Geometry check sheet. Reference: the model listing, model coordinates, mm. Face numbers are marked on the shaded views. A direction names the side the tool comes from. Give positions to 0.01 mm unless a question says otherwise; leave off trailing zeros. Order: outer loops, then holes, each group sorted by start corner. A loop starts at its lowest first (then second) coordinate and runs counter-clockwise, first axis right, second up. Notation, with made-up numbers: M -19,2 L -2,2 A7 cw -2,11 Z; hole C 1.25,26.25 d3. An arc over 180 degrees is marked long. Put each result on its own line as item: value. Start each with the question number.
Q1. Mould release check, pull along X, two halves, no side actions. Record for the marked faces 1, 2 and 3: +X half, -X half, draft (parallel to the pull), parting line (faces both ways), or undercut.
Q2. Material ranges on L1, parallel to Y at x = -0.5, z = -0.7; L2, parallel to Y at x = 0.25, z = 1.75; L3, parallel to X at y = 4, z = 0.65, recorded low to high.
Q3. Access from +Z, -Z, +X, -X, +Y, -Y to the whole of each face (thin tool, end or side, straight path). Record for the marked faces 4 and 5.
Q4. Section check C-C on x = 0. Record the cut outline in (y, z), then the cut area to 3 significant figures.
Q5. Go/stop test with flat-tipped pins: pin 1 (2 mm diameter, centred on x = -1, y = 45.5, fed in from -Z); pin 2 (2 mm diameter, centred on x = -0.34, y = 45, fed in from -Z). Record where each tip stops, or that it passes through.
Q6. Section check D-D on z = -2.05. Record the cut outline in (x, y).
Q7. Section check A-A on y = 25. Record the cut outline in (x, z).
Q8. Section check B-B on z = 0.9. Record the cut outline in (x, y).
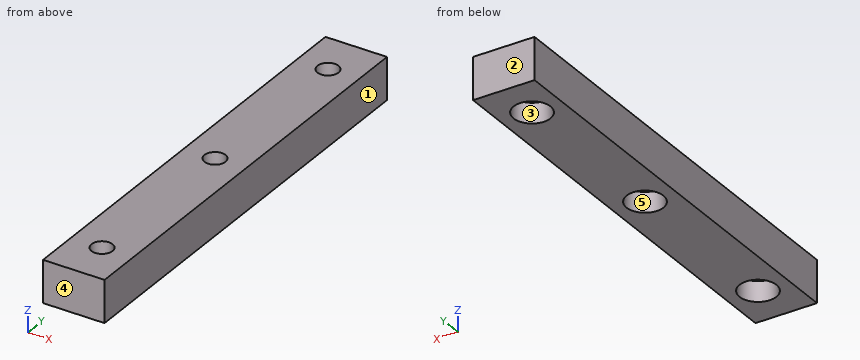
Autodesk Inventor part; units mm, degrees
ref_plane "YZ Plane" through (0, 0, 0) normal (1, 0, 0) x (0, 1, 0)
ref_plane "XZ Plane" through (0, 0, 0) normal (0, 1, 0) x (-1, 0, 0)
ref_plane "XY Plane" through (0, 0, 0) normal (0, 0, 1) x (1, 0, 0)
sketch "Sketch1" plane through (0, 0, 0) normal (0, 1, 0) x (-1, 0, 0)
  line L0 (3.8413, -2.6197) -> (-3.1587, -2.6197)
  line L1 (-3.1587, -2.6197) -> (-3.1587, 2.1803)
  line L2 (-3.1587, 2.1803) -> (3.8413, 2.1803)
  line L3 (3.8413, 2.1803) -> (3.8413, -2.6197)
  point P0 (0, 0)
  dimension "d0" = 4.8
  dimension "d1" = 7
extrude "Extrusion1" add sketch "Sketch1" along normal blind 50
sketch "Sketch2" plane through (3.1587, 0, -2.6197) normal (0, 0, -1) x (-1, 0, 0)
  circle A0 centre (3.5, 5) radius 1.2
  line L0 (0, 0) -> (7, 0)
  line L1 (7, 0) -> (7, 50)
  circle A1 centre (3.5, 25) radius 1.2
  circle A2 centre (3.5, 45) radius 1.2
  point P0 (3.1587, 0)
  dimension "d4" = 2.4
  dimension "d5" = 5
  dimension "d6" = 3.5
  dimension "d9" = 20
extrude "Extrusion2" cut sketch "Sketch2" against normal through all
sketch "Sketch3" plane through (3.1587, 0, -2.6197) normal (0, 0, -1) x (-1, 0, 0)
  circle A0 centre (3.5, 45) radius 1.2
  circle A1 centre (3.5, 45) radius 2.1
  circle A2 centre (3.5, 25) radius 1.2
  circle A3 centre (3.5, 25) radius 2.1
  circle A4 centre (3.5, 5) radius 1.2
  circle A5 centre (3.5, 5) radius 2.1
  point P0 (3.1587, 0)
  dimension "d16" = 4.2
  dimension "d17" = 4.2
  dimension "d18" = 4.2
extrude "Extrusion3" cut sketch "Sketch3" against normal blind 2.3 contours A0 | A1 | A2 | A3 | A4 | A5
properties part number "MGN7c_50mm_rail"
Results found:
1. face 1: +X half
1. face 2: draft
1. face 3: undercut
2. L1: y = 0 to 2.91, 7.09 to 22.91, 27.09 to 42.91, 47.09 to 50
2. L2: y = 0 to 3.96, 6.04 to 23.96, 26.04 to 43.96, 46.04 to 50
2. L3: x = -3.84 to -1, 0.32 to 3.16
3. face 4: +Z, -Z, +X, -X, -Y
3. face 5: -Z
4. outline: M 0,-2.62 L 2.93,-2.62 L 2.93,-0.32 L 3.85,-0.32 L 3.85,2.18 L 0,2.18 Z; M 6.15,-0.32 L 7.07,-0.32 L 7.07,-2.62 L 22.93,-2.62 L 22.93,-0.32 L 23.85,-0.32 L 23.85,2.18 L 6.15,2.18 Z; M 26.15,-0.32 L 27.07,-0.32 L 27.07,-2.62 L 42.93,-2.62 L 42.93,-0.32 L 43.85,-0.32 L 43.85,2.18 L 26.15,2.18 Z; M 46.15,-0.32 L 47.07,-0.32 L 47.07,-2.62 L 50,-2.62 L 50,2.18 L 46.15,2.18 Z
4. area: 194 mm^2
5. pin 1: stops at z = -0.32
5. pin 2: passes through
6. outline: M -3.84,0 L 3.16,0 L 3.16,50 L -3.84,50 Z; hole C -0.34,5 d4.2; hole C -0.34,25 d4.2; hole C -0.34,45 d4.2
7. outline: M -3.84,-2.62 L -2.44,-2.62 L -2.44,-0.32 L -1.54,-0.32 L -1.54,2.18 L -3.84,2.18 Z; M 0.86,-0.32 L 1.76,-0.32 L 1.76,-2.62 L 3.16,-2.62 L 3.16,2.18 L 0.86,2.18 Z
8. outline: M -3.84,0 L 3.16,0 L 3.16,50 L -3.84,50 Z; hole C -0.34,5 d2.4; hole C -0.34,25 d2.4; hole C -0.34,45 d2.4
